Source: CAD feature listing. Evaluate the final solid. Frame: model axes, mm. A direction names the side the tool comes from. Give positions to 0.01 mm unless a question says otherwise; leave off trailing zeros. Order: outer loops, then holes, each group sorted by start corner. A loop starts at its lowest first (then second) coordinate and runs counter-clockwise, first axis right, second up. Notation, with made-up numbers: (73.25, 88.25) -> (115.25, 88.25) arc R31 ccw to (115.25, 119.25) -> close; hole circle Ø3 at (36, 70). An arc over 180 degrees is marked (long way). Use CSV: the item, a comma, the result in double quotes.
Autodesk Inventor part; units mm, degrees
ref_plane "YZ Plane" through (0, 0, 0) normal (1, 0, 0) x (0, 1, 0)
ref_plane "XZ Plane" through (0, 0, 0) normal (0, 1, 0) x (-1, 0, 0)
ref_plane "XY Plane" through (0, 0, 0) normal (0, 0, 1) x (1, 0, 0)
sketch "Sketch1" plane through (0, 0, 0) normal (0, 0, 1) x (1, 0, 0)
  line L0 (0, 0) -> (25.4, 0)
  line L1 (25.4, 0) -> (25.4, 25.4)
  line L2 (25.4, 25.4) -> (0, 25.4)
  line L3 (0, 25.4) -> (0, 0)
  line L4 (3.175, 3.175) -> (22.225, 3.175)
  line L5 (22.225, 3.175) -> (22.225, 22.225)
  line L6 (22.225, 22.225) -> (3.175, 22.225)
  line L7 (3.175, 22.225) -> (3.175, 3.175)
  dimension "d0" = 25.4
  dimension "d1" = 25.4
  dimension "d2" = 3.175
extrude "Extrusion1" add sketch "Sketch1" against normal blind 990.6
sketch "Sketch2" plane through (0, 0, -990.6) normal (-1, 0, 0) x (0, 0, 1)
  line L0 (990.6, 25.4) -> (990.6, 0)
  line L1 (990.6, 0) -> (0, 0)
  line L2 (0, 25.4) -> (0, 0)
  line L3 (990.6, 25.4) -> (0, 25.4)
  point P0 (965.2, 12.7)
  point P1 (787.4, 12.7)
  point P2 (431.8, 12.7)
  point P3 (76.2, 12.7)
  point P4 (673.1, 12.7)
  point P5 (647.7, 12.7)
  point P6 (622.3, 12.7)
  point P7 (342.9, 12.7)
  point P8 (317.5, 12.7)
  point P9 (292.1, 12.7)
  point P10 (787.4, 12.7)
  point P11 (546.1, 12.7)
  point P12 (177.8, 12.7)
  point P13 (863.6, 12.7)
  point P14 (12.7, 12.7)
  point P15 (38.1, 12.7)
  dimension "d33" = 317.5
  dimension "d34" = 25.4
  dimension "d35" = 25.4
  dimension "d36" = 279.4
  dimension "d37" = 25.4
  dimension "d38" = 25.4
  dimension "d46" = 114.3
  dimension "d47" = 76.2
  dimension "d48" = 12.7
  dimension "d49" = 114.3
  dimension "d50" = 127
  dimension "d51" = 12.7
  dimension "d52" = 25.4
  dimension "d53" = 12.7
sketch "Sketch3" plane through (0, 0, 0) normal (0, -1, 0) x (1, 0, 0)
  line L0 (0, 0) -> (25.4, 0)
  point P0 (12.7, -12.7)
  point P1 (12.7, -38.1)
  dimension "d24" = 25.4
  dimension "d25" = 12.7
hole "Hole3" at (12.7, 0, -12.7) at (12.7, 0, -38.1) direction (0, 1, 0) diameter 6.35 depth 25.4 tip angle 118
hole "Hole4" at (0, 12.7, -317.5) at (0, 12.7, -342.9) at (0, 12.7, -368.3) at (0, 12.7, -647.7) at (0, 12.7, -673.1) at (0, 12.7, -698.5) at (0, 12.7, -444.5) at (0, 12.7, -812.8) at (0, 12.7, -127) direction (1, 0, 0) diameter 6.35 depth 25.4 tip angle 118
hole "Hole5" at (0, 12.7, -25.4) at (0, 12.7, -203.2) at (0, 12.7, -558.8) at (0, 12.7, -977.9) at (0, 12.7, -952.5) direction (1, 0, 0) diameter 6.35 depth 25.4 tip angle 118
properties part number "towertallbackthing"
1. Pin query (flat end, axial travel): P1, Ø5.5, axis at y = 12.7, z = -558.8, coming from the +X side; P2, Ø8.5, axis at x = 12.7, z = -12.7, coming from the -Y side. Return the tip coordinate at first contact, or that it passes through.
Answer below:
P1,"passes through"
P2,"stops at y = 0"
2. Mould query, pull axis Y, two halves, no side actions, for faces 3 (the flat face through (13, 0, -488)), 4 (the flat face through (13, 22.225, -488)), 5 (the flat face through (24, 13, -990.6)), 6 (the flat face through (13, 25.4, -488)). Classes: released by +Y, released by -Y, zero draft, split by the parting line, or undercut.
Answer below:
face 3,"released by -Y"
face 4,"undercut"
face 5,"zero draft"
face 6,"released by +Y"
3. Ray query, line 1 along Z through (x, y) = (13.75, 1.5); line 2 along Z through (x, y) = (12.7, 24.3) (3 decimals); line 3 along Y through (x, z) = (24.75, -558.8) (3 decimals). Return the intervals inside material, ascending.
Answer below:
line 1,"z = -990.6 to -41.1, -35.1 to -15.7, -9.7 to 0"
line 2,"z = -990.6 to -41.275, -34.925 to -15.875, -9.525 to 0"
line 3,"y = 0 to 9.525, 15.875 to 25.4"
4. Section query A-A on z = -602.5. Return loops of the section in (x, y) (3 decimals).
Answer below:
outline,"(0, 0) -> (25.4, 0) -> (25.4, 25.4) -> (0, 25.4) -> close; hole (3.175, 3.175) -> (22.225, 3.175) -> (22.225, 22.225) -> (3.175, 22.225) -> close"
5. Access query for faces 1 (the flat face through (0, 13, -488)), 2 (the flat face through (3.175, 13, -488)). Directions: +Z, -Z, +X, -X, +Y, -Y. A direction counts if a zero-diameter tool reaches every point of the face in a straight line with its end or side. Return the directions, or none.
Answer below:
face 1,"+Z, -Z, -X, +Y, -Y"
face 2,"+Z, -Z"
